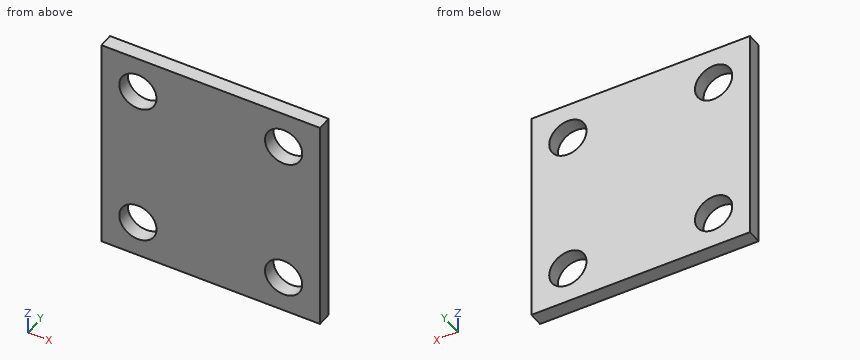
```python
from build123d import *

# Parameters (mm, degrees)
SKETCH1_W           = 38.1
SKETCH1_H           = 38.1
SKETCH1_R           = 3.25
BOSS_EXTRUDE1_DEPTH = 2.5


with BuildPart() as part:
    # Sketch1 → Boss-Extrude1 (new body)
    with BuildSketch(Plane(origin=(0, 0, 0), x_dir=(1, 0, 0), z_dir=(0, 1, 0))):
        Rectangle(SKETCH1_W, SKETCH1_H)
        with Locations((-12.7, 12.7)):
            Circle(SKETCH1_R, mode=Mode.SUBTRACT)
        with Locations((12.7, 12.7)):
            Circle(SKETCH1_R, mode=Mode.SUBTRACT)
        with Locations((-12.7, -12.7)):
            Circle(SKETCH1_R, mode=Mode.SUBTRACT)
        with Locations((12.7, -12.7)):
            Circle(SKETCH1_R, mode=Mode.SUBTRACT)
    extrude(amount=BOSS_EXTRUDE1_DEPTH)


solid = part.part
```
The listing builds one solid part. Answer for the finished solid, in the listing's coordinates (mm). Round coordinates to 2 decimals unless told otherwise and drop trailing zeros. Write each loop counter-clockwise with the first axis right and the second up, starting at its lowest first coordinate (ties: lowest second). Pieces come first, ordered by that corner, then holes. Notation, with made-up numbers: (-6, -15) -> (35, -15) arc R19 cw to (35, 10) -> close; hole circle Ø11 at (81, -33.5). An arc over 180 degrees is marked (long way). Answer as a JSON object with one key per item and string values. Group by question number.
Q1. Section C-C (z = 12.7) is taken. Write down the section's boundary in (x, y).
Q2. Straight lines are drawn through the part: line 1 along X through (y, z) = (0.75, -12.5); line 2 along Z through (x, y) = (12.7, 1); line 3 along X through (y, z) = (1.9, 10). For each, find the intervals that lie inside material, in ascending order.
Q3. Section B-B (y = 0.5) is taken. Write down the section's boundary in (x, z).
Q4. Section A-A (x = -12.7) is taken. Write down the section's boundary in (y, z).
Check values:
{
 "1": {"outline": "(-19.05, 0) -> (-15.95, 0) -> (-15.95, 2.5) -> (-19.05, 2.5) -> close; (-9.45, 0) -> (9.45, 0) -> (9.45, 2.5) -> (-9.45, 2.5) -> close; (15.95, 0) -> (19.05, 0) -> (19.05, 2.5) -> (15.95, 2.5) -> close"},
 "2": {"line 1": "-19.05 to -15.94, -9.46 to 9.46, 15.94 to 19.05", "line 2": "-19.05 to -15.95, -9.45 to 9.45, 15.95 to 19.05", "line 3": "-19.05 to -14.51, -10.89 to 10.89, 14.51 to 19.05"},
 "3": {"outline": "(-19.05, -19.05) -> (19.05, -19.05) -> (19.05, 19.05) -> (-19.05, 19.05) -> close; hole circle Ø6.5 at (-12.7, -12.7); hole circle Ø6.5 at (-12.7, 12.7); hole circle Ø6.5 at (12.7, -12.7); hole circle Ø6.5 at (12.7, 12.7)"},
 "4": {"outline": "(0, -19.05) -> (2.5, -19.05) -> (2.5, -15.95) -> (0, -15.95) -> close; (0, -9.45) -> (2.5, -9.45) -> (2.5, 9.45) -> (0, 9.45) -> close; (0, 15.95) -> (2.5, 15.95) -> (2.5, 19.05) -> (0, 19.05) -> close"}
}
